from build123d import *

# Parameters (mm, degrees)
SKETCH1_R           = 22.5
BOSS_EXTRUDE1_DEPTH = 1.984375
FILLET1_R           = 0.25
FILLET2_R           = 0.5


with BuildPart() as part:
    # Sketch1 → Boss-Extrude1 (new body)
    with BuildSketch(Plane.XY):
        with Locations((0, -0.070071084)):
            Circle(SKETCH1_R)
        with BuildLine():
            Line((-1.258126225, 20.778189514), (-0.928227613, 18.907241516))
            ThreePointArc((-0.928227613, 18.907241516), (3.299315376, 18.641276223), (7.362871814, 17.445296987))
            Line((7.362871814, 17.445296987), (8.312777007, 19.090581045))
            Line((8.312777007, 19.090581045), (12.437222993, 16.709331045))
            Line((12.437222993, 16.709331045), (11.487317799, 15.064046987))
            ThreePointArc((11.487317799, 15.064046987), (17.854159795, 6.428311639), (18.527819546, -4.279572584))
            Line((18.527819546, -4.279572584), (20.313057348, -4.929346005))
            Line((20.313057348, -4.929346005), (18.684186415, -9.404632111))
            Line((18.684186415, -9.404632111), (16.898948613, -8.75485869))
            ThreePointArc((16.898948613, -8.75485869), (14.554844419, -12.283035668), (11.487317799, -15.204189155))
            Line((11.487317799, -15.204189155), (12.437222993, -16.849473212))
            Line((12.437222993, -16.849473212), (8.312777007, -19.230723212))
            Line((8.312777007, -19.230723212), (7.362871814, -17.585439155))
            ThreePointArc((7.362871814, -17.585439155), (-3.299315376, -18.781418391), (-12.909445009, -14.010882737))
            Line((-12.909445009, -14.010882737), (-14.364784199, -15.232057315))
            Line((-14.364784199, -15.232057315), (-17.42606019, -11.583770655))
            Line((-17.42606019, -11.583770655), (-15.970721, -10.362596077))
            ThreePointArc((-15.970721, -10.362596077), (-17.854159795, -6.568453807), (-18.850189613, -2.451321084))
            Line((-18.850189613, -2.451321084), (-20.75, -2.451321084))
            Line((-20.75, -2.451321084), (-20.75, 2.311178916))
            Line((-20.75, 2.311178916), (-18.850189613, 2.311178916))
            ThreePointArc((-18.850189613, 2.311178916), (-14.554844419, 12.1428935), (-5.618374537, 18.080242069))
            Line((-5.618374537, 18.080242069), (-5.948273148, 19.951190068))
            Line((-5.948273148, 19.951190068), (-1.258126225, 20.778189514))
        make_face(mode=Mode.SUBTRACT)
        Polygon((20.377631163, 7.473973659), (21.19206663, 5.236330606), (20.487297164, 4.979815499), (19.672861698, 7.217458552), (18.858426231, 9.455101605), (19.563195697, 9.711616713), align=None, mode=Mode.SUBTRACT)
        Polygon((-14.55629531, 15.25261205), (-15.130828642, 15.734702757), (-16.661466638, 13.910559427), (-18.192104633, 12.086416097), (-17.617571301, 11.604325389), (-16.086933305, 13.428468719), align=None, mode=Mode.SUBTRACT)
        Polygon((-3.716164525, -21.384533086), (-6.061237987, -20.971033363), (-5.931001854, -20.232427548), (-3.585928392, -20.645927271), (-1.24085493, -21.059426994), (-1.371091064, -21.798032809), align=None, mode=Mode.SUBTRACT)
    extrude(amount=BOSS_EXTRUDE1_DEPTH)

    # Fillet1
    fillet1_edges = [part.edges().sort_by_distance(p)[0] for p in [
        (-18.850189613, -2.451321084, 0.9921875),
        (-15.970721, -10.362596077, 0.9921875),
        (-12.909445009, -14.010882737, 0.9921875),
        (7.362871814, -17.585439155, 0.9921875),
        (11.487317799, -15.204189155, 0.9921875),
        (16.898948613, -8.75485869, 0.9921875),
        (18.527819546, -4.279572584, 0.9921875),
        (11.487317799, 15.064046987, 0.9921875),
        (7.362871814, 17.445296987, 0.9921875),
        (-0.928227613, 18.907241516, 0.9921875),
        (-5.618374537, 18.080242069, 0.9921875),
        (-18.850189613, 2.311178916, 0.9921875),
    ]]
    fillet(fillet1_edges, radius=FILLET1_R)

    # Fillet2
    fillet2_edges = [part.edges().sort_by_distance(p)[0] for p in [
        (-17.42606019, -11.583770655, 0.9921875),
        (-14.364784199, -15.232057315, 0.9921875),
        (8.312777007, -19.230723212, 0.9921875),
        (12.437222993, -16.849473212, 0.9921875),
        (18.684186415, -9.404632111, 0.9921875),
        (20.313057348, -4.929346005, 0.9921875),
        (12.437222993, 16.709331045, 0.9921875),
        (8.312777007, 19.090581045, 0.9921875),
        (-1.258126225, 20.778189514, 0.9921875),
        (-5.948273148, 19.951190068, 0.9921875),
        (-20.75, 2.311178916, 0.9921875),
        (-20.75, -2.451321084, 0.9921875),
    ]]
    fillet(fillet2_edges, radius=FILLET2_R)


solid = part.part
The model under review builds one solid part; all positions refer to its coordinate system, in mm. A direction names the side the tool comes from. Round coordinates to 2 decimals unless told otherwise and drop trailing zeros. Write each loop counter-clockwise with the first axis right and the second up, starting at its lowest first coordinate (ties: lowest second). Pieces come first, ordered by that corner, then holes. Notation, with made-up numbers: M 84.25,60 L 121.25,60 A21 ccw 121.25,99 Z; hole C 13,54 d3. An arc over 180 degrees is marked long. Use a Markdown table: item, result. Add a question column.
Q1. Machinability: for faces 1 (the face through (19.281, -4.554, 0.978)), 2 (the face through (-12, 15, 0)), which of the approach directions +Z, -Z, +X, -X, +Y, -Y give a long, thin tool a straight path to every point of the face, cutting with its end or side? Answer none if there is none.
Q2. We need section A-A, the plane x = 0. State the section outline as (y, z) points, plus the area to 3 significant figures.
Q3. The part is to be moulded in two halves that separate along X. For faces 3 (the face through (19.51, -7.14, 0.98)), 4 (the face through (-12, 15, 1.984)), say which applies: pulls with the +X half, pulls with the -X half, needs draft (parallel to the pull), parting line crosses it, or undercut.
Q4. We need section C-C, the plane z = 0.55. Count the separate pieces of the cut face and the enclosed holes in it, plus the area to 3 significant figures.
Q5. Insertion check: pin 1 (4 mm diameter, centred on x = -0.5, y = 16, fed in from -Z); pin 2 (1 mm diameter, centred on y = 9, z = 1, fed in from +X). Each pin has a flat end and moves straight along its axis. Give the tip position at first contact, or say it passes through.
Q6. We need section B-B, the plane y = -12.5. State the section outline as (x, z) points.
Q7. To check wall thickness, follow line 1 (Y direction, x = -5, z = 0.8); line 2 (Y direction, x = -15, z = 1.9); line 3 (X direction, y = 6, z = 0.8). State the ranges of each line that lie inside material, in increasing order.
Findings below:
| question | item | result |
|---|---|---|
| 1 | face 1 | +Z, -Z |
| 1 | face 2 | -Z, +X, -X, +Y, -Y |
| 2 | outline | M -22.57,0 L -19.07,0 L -19.07,1.98 L -22.57,1.98 Z; M 18.93,0 L 22.43,0 L 22.43,1.98 L 18.93,1.98 Z |
| 2 | area | 13.9 mm² |
| 3 | face 3 | undercut |
| 3 | face 4 | needs draft |
| 4 | separate pieces | 1 |
| 4 | enclosed holes | 4 |
| 4 | area | 395 mm² |
| 5 | pin 1 | passes through |
| 5 | pin 2 | stops at x = 20.8 |
| 6 | outline | M -18.75,0 L -16.66,0 L -16.66,1.98 L -18.75,1.98 Z; M 14.37,0 L 18.75,0 L 18.75,1.98 L 14.37,1.98 Z |
| 7 | line 1 | y = -22.01 to -21.16, -20.4 to -18.4, 20.12 to 21.87 |
| 7 | line 2 | y = -16.84 to -14.48, 11.59 to 14.72, 15.62 to 16.7 |
| 7 | line 3 | x = -21.67 to -18, 18 to 20.12, 20.91 to 21.67 |
